Design review of the part built by this model. Coordinates are the model's own, in mm. Face numbers are marked on the shaded views. A direction names the side the tool comes from. Coordinates: 2 decimals unless noted, no trailing zeros. Order: outer loops, then holes, each group sorted by start corner. A loop starts at its lowest first (then second) coordinate and runs counter-clockwise, first axis right, second up. Notation, with made-up numbers: (22, 52) -> (36, 52) arc R24 ccw to (36, 68) -> close; hole circle Ø1 at (-19.75, 35). An arc over 180 degrees is marked (long way). Write item = value, one per line.
```python
from build123d import *

# Parameters (mm, degrees)
F0_W        = 177.8
F0_H        = 108.4261015058
F1_DEPTH    = 101.6
F2_R        = 50.7821410518
F3_DEPTH    = 76.2
F6_T        = 2.54
F6_T3_DEPTH = 15.513104752
F6_T5_DEPTH = 105.7102081755
F7_R        = 45.225137574
F8_DEPTH    = 50.8


# Not quite as in the source:
# - a feature of the source that left no trace in its solid (it failed there, or was rolled back) is left out
# - a shell that OpenCascade refuses in one call is made with other operations: the cavity is built on its own and cut out


with BuildPart() as f1:
    # F0 (on Top) → F1 (new body)
    with BuildSketch(Plane.XY):
        with Locations((-74.0991531372, 54.2130507529)):
            Rectangle(F0_W, F0_H)
    extrude(amount=F1_DEPTH)

    # F2 (on face) → F3 (join)
    with BuildSketch(Plane(origin=(0, 108.4261015058, 0), x_dir=(-1, 0, 0), z_dir=(0, 1, 0))):
        with Locations((-14.0330018476, 49.8538725078)):
            Circle(F2_R)
    extrude(amount=F3_DEPTH)

    # F6: shell of thickness 2.54, made by hand


with BuildPart() as f6_core1:
    # F6_t2: copy of F1
    add(f1.part)

    # the walls: a layer under each face that stays
    f6_faces = [f6_core1.faces().sort_by_distance(p)[0] for p in [
        (64.8151428994, 146.5261015058, 49.8538725078),
        (-74.0991531372, 54.2130507529, 0),
        (-162.9991531372, 54.2130507529, 50.8),
        (-74.0991531372, 54.2130507529, 101.6),
        (14.8008468628, 54.2130507529, 50.8),
        (34.5914425051, 108.4261015058, 49.8509698158),
    ]]
    thicken(f6_faces, amount=-F6_T, mode=Mode.SUBTRACT)

    # F6_s4 → F6_t3 (cut)
    with BuildSketch(Plane.YZ.offset(1.8277421108)):
        Polygon((108.4007015058, -0.0254), (108.4261015058, 2.54), (110.9661015058, 2.54), (110.9661015058, 0), align=None)
    extrude(amount=F6_T3_DEPTH, mode=Mode.SUBTRACT)

    # F6_s6 → F6_t5 (cut)
    with BuildSketch(Plane.XY.offset(-2.54)):
        Polygon((14.8262468628, 108.4007015058), (12.2608468628, 108.4261015058), (12.2608468628, 110.9661015058), (14.8008468628, 110.9661015058), align=None)
    extrude(amount=F6_T5_DEPTH, mode=Mode.SUBTRACT)


with BuildPart() as f1_1:
    add(f1.part)

    # what is left inside the walls is the cavity
    f6_cavity = [f6_core1.part.solids().sort_by_distance(p)[0] for p in [
        (62.249743, 159.226102, 49.853873),
    ]]
    add(f6_cavity, mode=Mode.SUBTRACT)

    # F7 (on face) → F8 (cut)
    with BuildSketch(Plane(origin=(0, 0, 0), x_dir=(1, 0, 0), z_dir=(0, 0, -1))):
        with Locations((-6.2627755105, -46.561319381)):
            Circle(F7_R)
    extrude(amount=-F8_DEPTH, mode=Mode.SUBTRACT)


solid = f1_1.part
```
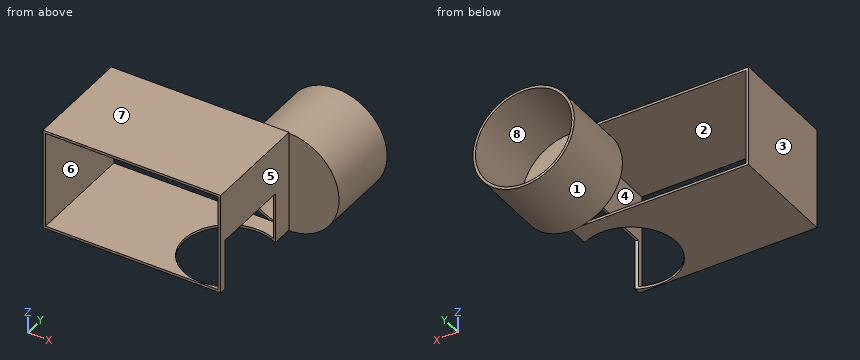
(1) The part is to be moulded in two halves that separate along Z. For the marked faces 1, 2, 3 and 4, say which applies: released by +Z, released by -Z, zero draft, split by the parting line, or undercut.
Report:
face_1 = split by the parting line
face_2 = undercut
face_3 = zero draft
face_4 = undercut
(2) Insertion check: pin 1 (4 mm diameter, centred on x = -96, y = 77.5, fed in from -Z); pin 2 (4 mm diameter, centred on y = 52, z = 80.5, fed in from +X); pin 3 (5 mm diameter, centred on x = 18.5, y = 133, fed in from +Z); pin 4 (12 mm diameter, centred on x = -103.5, z = 13, fed in from +Y). Each pin has a flat end and moves straight along its axis. Give the tip position at first contact, or say it passes through.
Report:
pin_1 = 0
pin_2 = 14.8
pin_3 = 100.6
pin_4 = through
(3) We need section D-D (z = 65). Write out the cut boundary in (x, y), and give its area (3 significant figures).
Report:
outline = (-163, 0) -> (-160.46, 0) -> (-160.46, 108.43) -> (-163, 108.43) -> close; (-34.44, 108.43) -> (-31.77, 108.43) -> (-31.77, 184.63) -> (-34.44, 184.63) -> close; (12.26, 0) -> (14.8, 0) -> (14.8, 108.43) -> (62.5, 108.43) -> (62.5, 184.63) -> (59.84, 184.63) -> (59.84, 110.97) -> (12.26, 110.97) -> close
area = 1,080 mm²
(4) For the marked faces 5, 6, 7 and 8, list the 3-axis set-ups (+Z, -Z, +X, -X, +Y, -Y) from which the entire face can be reached by the end or side of a thin tool; tool diameter is ignored.
Report:
face_5 = +Z, -Z, +X, -Y
face_6 = +Y, -Y
face_7 = +Z, +X, -X, +Y, -Y
face_8 = +Y
(5) We need section C-C (x = -46.5). Write out the cut boundary in (y, z), and give its area (3 significant figures).
Report:
outline = (0, 0) -> (25.91, 0) -> (25.91, 2.54) -> (0, 2.54) -> close; (0, 99.06) -> (108.43, 99.06) -> (108.43, 101.6) -> (0, 101.6) -> close; (67.21, 0) -> (108.43, 0) -> (108.43, 2.54) -> (67.21, 2.54) -> close
area = 446 mm²
(6) We need section A-A (x = -78.5). Write out the cut boundary in (y, z).
Report:
outline = (0, 0) -> (108.43, 0) -> (108.43, 2.54) -> (0, 2.54) -> close; (0, 99.06) -> (108.43, 99.06) -> (108.43, 101.6) -> (0, 101.6) -> close
(7) For L1, parallel to X at y = 96, z = 63; L2, parallel to Z at x = -84, y = 91; L3, parallel to Z at x = -38, y = 44.5, list the stretches that pass through material, from the lowest coordinate up.
Report:
L1 = -163 to -160.46, 12.26 to 14.8
L2 = 0 to 2.54, 99.06 to 101.6
L3 = 99.06 to 101.6
(8) We need section B-B (z = 30). Write out the cut boundary in (x, y), and give its area (3 significant figures).
Report:
outline = (-163, 0) -> (-160.46, 0) -> (-160.46, 108.43) -> (-163, 108.43) -> close; (-32.71, 108.43) -> (-29.93, 108.43) -> (-29.93, 184.63) -> (-32.71, 184.63) -> close; (12.26, 0) -> (14.8, 0) -> (14.8, 6.54) arc R45.23 cw to (12.26, 5.3) -> close; (12.26, 87.82) arc R45.23 cw to (14.8, 86.58) -> (14.8, 108.43) -> (60.77, 108.43) -> (60.77, 184.63) -> (58, 184.63) -> (58, 110.97) -> (12.26, 110.97) -> close
area = 883 mm²
